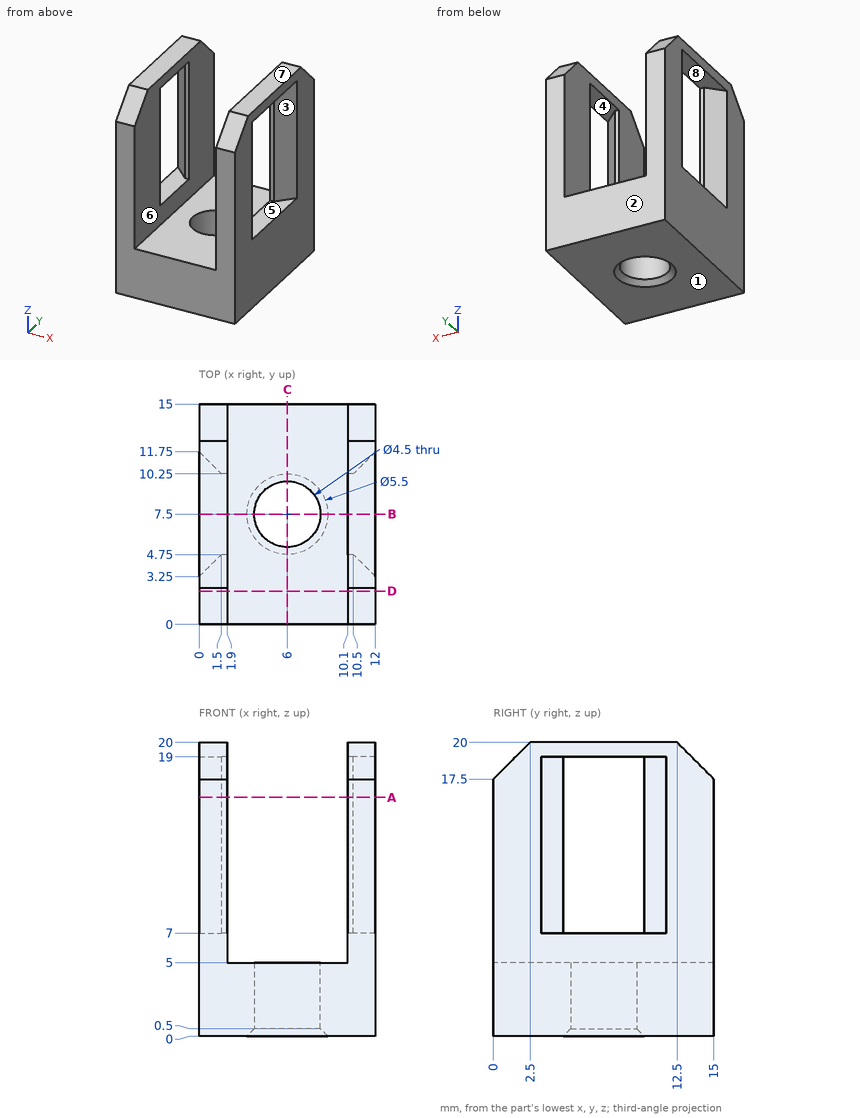
Design review of the part shown in the three views and the two pictorial views. Dimensions are in mm from the part's minimum x, y and z. A direction names the side the tool comes from. Coordinates: 2 decimals unless noted, no trailing zeros. Order: outer loops, then holes, each group sorted by start corner. A loop starts at its lowest first (then second) coordinate and runs counter-clockwise, first axis right, second up.
1) Take a section at A-A, the plane z = 16.25. Give the boundary of the cut face in (x, y), and give its area (3 significant figures).
2) Take a section at D-D, the plane y = 2.25. Give the boundary of the cut face in (x, z), and give its area (3 significant figures).
3) For the marked faces 5, 6, 7 and 8, list the 3-axis set-ups (+Z, -Z, +X, -X, +Y, -Y) from which the entire face can be reached by the end or side of a thin tool; tool diameter is ignored.
4) Take a section at B-B, the plane y = 7.5. Give the boundary of the cut face in (x, z), and give its area (4 significant figures).
5) Take a section at C-C, the plane x = 6. Give the boundary of the cut face in (y, z).
6) Mouldability with a two-part tool opening along Z and no side actions: class the marked faces 1, 2, 3 and 4 as +Z half, -Z half, draft (parallel to the pull), parting line (faces both ways), or undercut.
7) Clearance check with flat-ended pins moving along their axes: pin 1 (1 mm diameter, centred on x = 1, y = 7, fed in from -Z); pin 2 (6 mm diameter, centred on x = 6, y = 13, fed in from +Z). State where each tip first meets the part, or that it passes through.
8) Wall thickness on line 1 along X through (y, z) = (7.5, 2.8); line 2 along Y through (x, z) = (6, 3.1); line 3 along X through (y, z) = (10.25, 5.25): over which ranges is each line inside the solid? List them lowest first.
Returned:
1. outline: (0, 0) - (1.9, 0) - (1.9, 4.75) - (1.5, 4.75) - (0, 3.25) - close; (0, 11.75) - (1.5, 10.25) - (1.9, 10.25) - (1.9, 15) - (0, 15) - close; (10.1, 0) - (12, 0) - (12, 3.25) - (10.5, 4.75) - (10.1, 4.75) - close; (10.1, 10.25) - (10.5, 10.25) - (12, 11.75) - (12, 15) - (10.1, 15) - close
1. area: 31.6 mm2
2. outline: (0, 0) - (12, 0) - (12, 19.75) - (10.1, 19.75) - (10.1, 5) - (1.9, 5) - (1.9, 19.75) - (0, 19.75) - close
2. area: 116 mm2
3. face 5: +X
3. face 6: +Z, +Y, -Y
3. face 7: +Z, +X, -X, +Y, -Y
3. face 8: -X
4. outline: (0, 0) - (3.25, 0) - (3.75, 0.5) - (3.75, 5) - (1.9, 5) - (1.9, 7) - (0, 7) - close; (0, 19) - (1.9, 19) - (1.9, 20) - (0, 20) - close; (8.25, 0.5) - (8.75, 0) - (12, 0) - (12, 7) - (10.1, 7) - (10.1, 5) - (8.25, 5) - close; (10.1, 19) - (12, 19) - (12, 20) - (10.1, 20) - close
4. area: 48.65 mm2
5. outline: (0, 0) - (4.75, 0) - (5.25, 0.5) - (5.25, 5) - (0, 5) - close; (9.75, 0.5) - (10.25, 0) - (15, 0) - (15, 5) - (9.75, 5) - close
6. face 1: -Z half
6. face 2: draft
6. face 3: undercut
6. face 4: undercut
7. pin 1: stops at z = 0
7. pin 2: stops at z = 5
8. line 1: x = 0 to 3.75, 8.25 to 12
8. line 2: y = 0 to 5.25, 9.75 to 15
8. line 3: x = 0 to 1.9, 10.1 to 12
